Source: CAD feature listing. Evaluate the final solid. Frame: model axes, mm. A direction names the side the tool comes from. Round coordinates to 2 decimals unless told otherwise and drop trailing zeros. Loops run counter-clockwise (first coordinate to the right, second up) from the corner with the lowest first, then second, coordinate; pieces in that order, holes last.
(1) Material intervals for probe 1 along Y at (x, z) = (0, 5); probe 2 along X at (y, z) = (-3, 17.75); probe 3 along X at (y, z) = (-6, 19.25), sorted ascending.
(2) First-contact query: pin 1 Ø2 at (x, y) = (-4.5, 2.5) entering from +Z; pin 2 Ø2 at (x, y) = (-2, -2.5) entering from -Z; pin 3 Ø6 at (y, z) = (4.5, 12) entering from -X. Flat tips, straight axial feed; report the tip coordinate or a pass-through.
(3) Mould query, pull axis Z, two halves, no side actions, for faces 6 (the cylindrical face through (-3.019, -5.185, 15.972)), 7 (the flat face through (4, -3, 9)), 8 (the flat face through (4, 4, 15)). Classes: pulls with the +Z half, pulls with the -Z half, needs draft (parallel to the pull), parting line crosses it, or undercut.
(4) Section A-A, the plane z = 14.75. Return the cut outline in (x, y).
(5) Set-up query: faces 1 (the conical face through (3.115, 5.35, 18.191)), 2 (the flat face through (0, 5, 9)), 3 (the flat face through (4.93, -1.32, 14.58)), 4 (the flat face through (-1.33, -4.97, 14.58)), 5 (the conical face through (-3.115, -5.35, 18.191)). Return all of +Z, -Z, +X, -X, +Y, -Y with unobstructed straight access to the full face (end or side cutting, diameter ignored); none if empty.
(6) Section C-C, the plane z = 8.5. Return the cut outline in (x, y), plus the area to 3 significant figures.
(7) Section B-B, the plane z = 12.25. Return the cut outline in (x, y).
```python
from build123d import *

# Parameters (mm, degrees)
CYLINDER001_R      = 3.75
CYLINDER001_DEPTH  = 30
CYLINDER002_R      = 6
CYLINDER002_DEPTH  = 6
CYLINDER003_R      = 8
CYLINDER003_DEPTH  = 6
CHAMFER_SIZE       = 1
CYLINDER_R         = 6.5
CYLINDER_DEPTH     = 20
FILLET_R           = 2
CHAMFER001_SIZE    = 1
FILLET001_R        = 1
POCKET_DEPTH       = 11
POLARPATTERN_COUNT = 6
CHAMFER002_SIZE    = 0.5
FILLET002_R        = 1
CHAMFER003_SIZE    = 0.5


with BuildPart() as cilindro001:
    # Cylinder001 → Cylinder001 (new body)
    with BuildSketch(Plane.XY):
        Circle(CYLINDER001_R)
    extrude(amount=CYLINDER001_DEPTH)


with BuildPart() as cilindro002:
    # Cylinder002 → Cylinder002 (new body)
    with BuildSketch(Plane.XY):
        Circle(CYLINDER002_R)
    extrude(amount=CYLINDER002_DEPTH)


with BuildPart() as chamfer_body:
    # Cylinder003 → Cylinder003 (new body)
    with BuildSketch(Plane.XY):
        Circle(CYLINDER003_R)
    extrude(amount=CYLINDER003_DEPTH)

    # Cut: cut Cilindro002
    add(cilindro002.part, mode=Mode.SUBTRACT)


with BuildPart() as chamfer_body_1:
    # Cut placement: moved
    add(chamfer_body.part.moved(Location((0, 0, 13))))

    # Chamfer
    chamfer_edges = [chamfer_body_1.edges().sort_by_distance(p)[0] for p in [
        (-6, 0, 19),
        (-6, 0, 13),
    ]]
    chamfer(chamfer_edges, length=CHAMFER_SIZE)


with BuildPart() as chamfer003:
    # Cylinder → Cylinder (new body)
    with BuildSketch(Plane.XY):
        Circle(CYLINDER_R)
    extrude(amount=CYLINDER_DEPTH)

    # Cut001: cut Chamfer body
    add(chamfer_body_1.part, mode=Mode.SUBTRACT)

    # Cut002: cut Cilindro001
    add(cilindro001.part, mode=Mode.SUBTRACT)

    # Fillet
    fillet_edges = [chamfer003.edges().sort_by_distance(p)[0] for p in [
        (-3.75, 0, 20),
    ]]
    fillet(fillet_edges, radius=FILLET_R)

    # Chamfer001
    chamfer001_edges = [chamfer003.edges().sort_by_distance(p)[0] for p in [
        (-3.75, 0, 0),
    ]]
    chamfer(chamfer001_edges, length=CHAMFER001_SIZE)

    # Fillet001
    fillet001_edges = [chamfer003.edges().sort_by_distance(p)[0] for p in [
        (-3.75, 0, 1),
    ]]
    fillet(fillet001_edges, radius=FILLET001_R)

    # Sketch → Pocket (cut)
    with BuildSketch(Plane.XY.offset(20)):
        Polygon((0, 0), (-1.811733, 6.761481), (1.811733, 6.761481), align=None)
    pocket = extrude(amount=-POCKET_DEPTH, mode=Mode.SUBTRACT)

    # PolarPattern: Pocket ×6 about axis
    polarpattern_axis = Axis((0, 0, 20), (0, 0, 1))
    for i in range(1, POLARPATTERN_COUNT):
        add(pocket.rotate(polarpattern_axis, i * 360 / POLARPATTERN_COUNT), mode=Mode.SUBTRACT)

    # Chamfer002
    chamfer002_edges = [chamfer003.edges().sort_by_distance(p)[0] for p in [
        (3.25, -5.629165, 20),
        (-3.25, -5.629165, 20),
        (6.444392, 0.84842, 20),
        (6.444392, -0.84842, 20),
        (3.25, 5.629165, 20),
        (-3.25, 5.629165, 20),
        (-6.5, 0, 20),
    ]]
    chamfer(chamfer002_edges, length=CHAMFER002_SIZE)

    # Fillet002
    fillet002_edges = [chamfer003.edges().sort_by_distance(p)[0] for p in [
        (6.444392, 0.84842, 19.5),
        (6.444392, -0.84842, 19.5),
        (3.25, -5.629165, 19.5),
        (-3.25, -5.629165, 19.5),
        (3.25, 5.629165, 19.5),
        (-3.25, 5.629165, 19.5),
        (-6.5, 0, 19.5),
    ]]
    fillet(fillet002_edges, radius=FILLET002_R)

    # Chamfer003
    chamfer003_edges = [chamfer003.edges().sort_by_distance(p)[0] for p in [
        (-6.5, 0, 0),
    ]]
    chamfer(chamfer003_edges, length=CHAMFER003_SIZE)


solid = chamfer003.part
```
Output values:
1. probe 1: y = -6.5 to -3.75, 3.75 to 6.5
1. probe 2: x = -3 to -2.25, 2.25 to 3
1. probe 3: x = -2.46 to -1.61, 1.61 to 2.46
2. pin 1: stops at z = 9
2. pin 2: stops at z = 0.55
2. pin 3: stops at x = -6.32
3. face 6: undercut
3. face 7: pulls with the +Z half
3. face 8: needs draft
4. outline: (-5.8, -1.55) - (-3.62, -0.97) arc R3.75 cw to (-3.62, 0.97) - (-5.8, 1.55) arc R6 ccw to start; (-4.24, -4.24) arc R6 ccw to (-1.55, -5.8) - (-0.97, -3.62) arc R3.75 cw to (-2.65, -2.65) - close; (-4.24, 4.24) - (-2.65, 2.65) arc R3.75 cw to (-0.97, 3.62) - (-1.55, 5.8) arc R6 ccw to start; (0.97, -3.62) - (1.55, -5.8) arc R6 ccw to (4.24, -4.24) - (2.65, -2.65) arc R3.75 cw to start; (0.97, 3.62) arc R3.75 cw to (2.65, 2.65) - (4.24, 4.24) arc R6 ccw to (1.55, 5.8) - close; (3.62, -0.97) - (5.8, -1.55) arc R6 ccw to (5.8, 1.55) - (3.62, 0.97) arc R3.75 cw to start
5. face 1: +X, +Y
5. face 2: +Z, +Y
5. face 3: +Z
5. face 4: +Z, -Y
5. face 5: -X, -Y
6. outline: circle Ø13 at (0, 0); hole circle Ø7.5 at (0, 0)
6. area: 88.6 mm2
7. outline: (-6.28, -1.68) - (-3.62, -0.97) arc R3.75 cw to (-3.62, 0.97) - (-6.28, 1.68) arc R6.5 ccw to start; (-4.6, -4.6) arc R6.5 ccw to (-1.68, -6.28) - (-0.97, -3.62) arc R3.75 cw to (-2.65, -2.65) - close; (-4.6, 4.6) - (-2.65, 2.65) arc R3.75 cw to (-0.97, 3.62) - (-1.68, 6.28) arc R6.5 ccw to start; (0.97, -3.62) - (1.68, -6.28) arc R6.5 ccw to (4.6, -4.6) - (2.65, -2.65) arc R3.75 cw to start; (0.97, 3.62) arc R3.75 cw to (2.65, 2.65) - (4.6, 4.6) arc R6.5 ccw to (1.68, 6.28) - close; (3.62, -0.97) - (6.28, -1.68) arc R6.5 ccw to (6.28, 1.68) - (3.62, 0.97) arc R3.75 cw to start
